from build123d import *

# Parameters (mm, degrees)
SKETCH1_R               = 75
BOSS_EXTRUDE1_DEPTH     = 5
SKETCH2_R               = 14
SKETCH2_R_2             = 10
SKETCH2_R_3             = 4
BOSS_EXTRUDE2_DEPTH     = 25
SKETCH3_R               = 4
CUT_EXTRUDE1_DEPTH      = 12
CUT_EXTRUDE2_REACH      = 122.192
CUT_EXTRUDE2_END_RADIUS = 10
SKETCH4_R               = 1.5
CUT_EXTRUDE3_REACH      = 122.192
CUT_EXTRUDE3_END_RADIUS = 10
SKETCH5_R               = 1.5
SKETCH6_R               = 2
CUT_EXTRUDE4_DEPTH      = 111.227038452
SKETCH7_R               = 1.5
CUT_EXTRUDE5_DEPTH      = 111.227038452
CUT_EXTRUDE6_DEPTH      = 25
BOSS_EXTRUDE3_DEPTH     = 20
SKETCH10_R              = 1.5
CUT_EXTRUDE7_DEPTH      = 113.116290101
FILLET1_R               = 1


with BuildPart() as part:
    # Sketch1 → Boss-Extrude1 (new body)
    with BuildSketch(Plane(origin=(0, 0, 0), x_dir=(1, 0, 0), z_dir=(0, 1, 0))):
        with Locations(Location((0, 0, 0), (0, 0, 270))):
            Circle(SKETCH1_R)
    extrude(amount=BOSS_EXTRUDE1_DEPTH)

    # Sketch2 → Boss-Extrude2 (add)
    with BuildSketch(Plane(origin=(0, 5, 0), x_dir=(1, 0, 0), z_dir=(0, 1, 0))):
        with Locations(Location((0, 0, 0), (0, 0, 270))):
            Circle(SKETCH2_R)
        with Locations(Location((0, 0, 0), (0, 0, 270))):
            Circle(SKETCH2_R_2, mode=Mode.SUBTRACT)
        with Locations(Location((0, 0, 0), (0, 0, 270))):
            Circle(SKETCH2_R_3)
    extrude(amount=BOSS_EXTRUDE2_DEPTH)

    # Sketch3 → Cut-Extrude1 (cut)
    with BuildSketch(Plane(origin=(0, 30, 0), x_dir=(1, 0, 0), z_dir=(0, 1, 0))):
        with Locations(Location((0, 0, 0), (0, 0, 270))):
            Circle(SKETCH3_R)
    extrude(amount=-CUT_EXTRUDE1_DEPTH, mode=Mode.SUBTRACT)

    # Cut-Extrude2: up to this cylinder (the profile starts outside it)
    cut_extrude2_end = Plane(origin=(0, 8.4, 0), z_dir=(0, -1, 0)) * Cylinder(CUT_EXTRUDE2_END_RADIUS, 265.384, mode=Mode.PRIVATE)
    # Sketch4 → Cut-Extrude2 (cut, up to the surface)
    with BuildSketch(Plane(origin=(14, 0, 0), x_dir=(0, 0, -1), z_dir=(1, 0, 0)), mode=Mode.PRIVATE) as cut_extrude2_sk1:
        with Locations((-1, 8.4)):
            Circle(SKETCH4_R)
    cut_extrude2_tool1 = extrude(cut_extrude2_sk1.sketch, amount=-CUT_EXTRUDE2_REACH, mode=Mode.PRIVATE) - cut_extrude2_end
    add(cut_extrude2_tool1.solids().sort_by_distance((14, 8.4, 1))[0], mode=Mode.SUBTRACT)

    # Cut-Extrude3: up to this cylinder (the profile starts outside it)
    cut_extrude3_end = Plane(origin=(0, 8.4, 0), z_dir=(0, -1, 0)) * Cylinder(CUT_EXTRUDE3_END_RADIUS, 265.384, mode=Mode.PRIVATE)
    # Sketch5 → Cut-Extrude3 (cut, up to the surface)
    with BuildSketch(Plane.XY.offset(14), mode=Mode.PRIVATE) as cut_extrude3_sk1:
        with Locations((-1, 8.4)):
            Circle(SKETCH5_R)
    cut_extrude3_tool1 = extrude(cut_extrude3_sk1.sketch, amount=-CUT_EXTRUDE3_REACH, mode=Mode.PRIVATE) - cut_extrude3_end
    add(cut_extrude3_tool1.solids().sort_by_distance((-1, 8.4, 14))[0], mode=Mode.SUBTRACT)

    # Sketch6 → Cut-Extrude4 (cut, through all)
    with BuildSketch(Plane.XZ):
        with Locations(Location((-18, 0, 0), (0, 0, 270))):
            Circle(SKETCH6_R)
        with Locations(Location((18, 0, 0), (0, 0, 270))):
            Circle(SKETCH6_R)
    extrude(amount=-CUT_EXTRUDE4_DEPTH, mode=Mode.SUBTRACT)

    # Sketch7 → Cut-Extrude5 (cut, through all)
    with BuildSketch(Plane.XZ):
        with Locations(Location((20, 47.5, 0), (0, 0, 270))):
            Circle(SKETCH7_R)
        with Locations(Location((33, 47.5, 0), (0, 0, 270))):
            Circle(SKETCH7_R)
        with Locations(Location((20, 25.5, 0), (0, 0, 270))):
            Circle(SKETCH7_R)
        with Locations(Location((33, 25.5, 0), (0, 0, 270))):
            Circle(SKETCH7_R)
        with Locations(Location((-20, 25.5, 0), (0, 0, 270))):
            Circle(SKETCH7_R)
        with Locations(Location((-33, 25.5, 0), (0, 0, 270))):
            Circle(SKETCH7_R)
        with Locations(Location((-33, 47.5, 0), (0, 0, 270))):
            Circle(SKETCH7_R)
        with Locations(Location((-20, 47.5, 0), (0, 0, 270))):
            Circle(SKETCH7_R)
        with Locations(Location((-33, -47.5, 0), (0, 0, 270))):
            Circle(SKETCH7_R)
        with Locations(Location((-20, -47.5, 0), (0, 0, 270))):
            Circle(SKETCH7_R)
        with Locations(Location((-20, -25.5, 0), (0, 0, 270))):
            Circle(SKETCH7_R)
        with Locations(Location((-33, -25.5, 0), (0, 0, 270))):
            Circle(SKETCH7_R)
        with Locations(Location((20, -25.5, 0), (0, 0, 270))):
            Circle(SKETCH7_R)
        with Locations(Location((20, -47.5, 0), (0, 0, 270))):
            Circle(SKETCH7_R)
        with Locations(Location((33, -47.5, 0), (0, 0, 270))):
            Circle(SKETCH7_R)
        with Locations(Location((33, -25.5, 0), (0, 0, 270))):
            Circle(SKETCH7_R)
    extrude(amount=-CUT_EXTRUDE5_DEPTH, mode=Mode.SUBTRACT)

    # Sketch8 → Cut-Extrude6 (cut)
    with BuildSketch(Plane(origin=(0, 30, 0), x_dir=(1, 0, 0), z_dir=(0, 1, 0))):
        with BuildLine():
            Line((0.75, 13.97989628), (0.75, 9.971835338))
            ThreePointArc((0.75, 9.971835338), (0, 10), (-0.75, 9.971835338))
            Line((-0.75, 9.971835338), (-0.75, 13.97989628))
            ThreePointArc((-0.75, 13.97989628), (0, 14), (0.75, 13.97989628))
        make_face()
    extrude(amount=-CUT_EXTRUDE6_DEPTH, mode=Mode.SUBTRACT)

    # Sketch9 → Boss-Extrude3 (add)
    with BuildSketch(Plane(origin=(0, 30, 0), x_dir=(1, 0, 0), z_dir=(0, 1, 0))):
        with BuildLine():
            Line((0.75, 13.97989628), (0.75, 21.727253913))
            Line((0.75, 21.727253913), (2.75, 21.727253913))
            Line((2.75, 21.727253913), (2.75, 13.727253913))
            ThreePointArc((2.75, 13.727253913), (1.754553231, 13.889619972), (0.75, 13.97989628))
        make_face()
        with BuildLine():
            Line((-0.75, 21.727253913), (-2.75, 21.727253913))
            Line((-2.75, 21.727253913), (-2.75, 13.727253913))
            ThreePointArc((-2.75, 13.727253913), (-1.754553231, 13.889619972), (-0.75, 13.97989628))
            Line((-0.75, 13.97989628), (-0.75, 21.727253913))
        make_face()
    extrude(amount=-BOSS_EXTRUDE3_DEPTH)

    # Sketch10 → Cut-Extrude7 (cut, through all)
    with BuildSketch(Plane(origin=(2.75, 0, 0), x_dir=(0, 0, -1), z_dir=(1, 0, 0))):
        with Locations(Location((17.727253913, 24, 0), (0, 0, 180))):
            Circle(SKETCH10_R)
        with Locations(Location((17.727253913, 16, 0), (0, 0, 180))):
            Circle(SKETCH10_R)
    extrude(amount=-CUT_EXTRUDE7_DEPTH, mode=Mode.SUBTRACT)

    # Fillet1
    fillet1_edges = [part.edges().sort_by_distance(p)[0] for p in [
        (13.994973168, 5, 0.375134696),
    ]]
    fillet(fillet1_edges, radius=FILLET1_R)


solid = part.part
Can you work these out from the model? Positions are in its coordinate system, mm. A direction names the side the tool comes from. Round coordinates to 2 decimals unless told otherwise and drop trailing zeros. Write each loop counter-clockwise with the first axis right and the second up, starting at its lowest first coordinate (ties: lowest second). Pieces come first, ordered by that corner, then holes. Notation, with made-up numbers: (25, 31) - (39, 31) arc R18 cw to (39, 52) - close; hole circle Ø2 at (31.25, 78). An arc over 180 degrees is marked (long way). Write each question's results on one line, items separated by ' | '. Start each with the question number.
1) Please list where these lines run through material, in increasing order: line 1 (X direction, y = 1.5, z = 0); line 2 (Z direction, x = -1, y = 16); line 3 (X direction, y = 28.5, z = -16).
2) We'd pull the mould along X, two halves only. Please class faces 4 (the flat face through (-0.75, 20, -16)), 5 (the flat face through (2.75, 20, -18)), 6 (the flat face through (-1, 30, -11)): released by +X, released by -X, zero draft, split by the parting line, or undercut.
3) Suppose I cut it at D-D (z = -42). List the corners of the cut face in (x, y) for me.
4) For pin 1 Ø6 at (y, z) = (15.5, -15.5) entering from +X; pin 2 Ø2.5 at (x, z) = (18, 0) entering from -Y; pin 3 Ø2.5 at (x, y) = (-1, 8.4) entering from +Z; pin 4 Ø4 at (y, z) = (24, -17.73) entering from -X, each with a flat end and sliding along its axis, tell me the tip position at first contact or that it passes through.
5) Suppose I cut it at C-C (x = 59). List the corners of the cut face in (y, z) for me.
6) Which directions (+Z, -Z, +X, -X, +Y, -Y) give clear straight access to the entire face, cutting with the end or side of a thin tool? Please do faces 1 (the cylindrical face through (-3.905, 11.409, -0.867)), 2 (the flat face through (-2.75, 20, -18)), 3 (the flat face through (0.75, 20, -16)).
7) Suppose I cut it at B-B (y = 27.5). List the corners of the cut face in (x, z) for me, and give its area (3 significant figures).
8) Suppose I cut it at A-A (y = 12.5). List the corners of the cut face in (x, z) for me.
Here are the results:
1) line 1: x = -75 to -20, -16 to 16, 20 to 75 | line 2: z = -21.73 to -19.23, -16.23 to -9.95, -3.87 to 3.87, 9.95 to 13.96 | line 3: x = -2.75 to -0.75, 0.75 to 2.75
2) face 4: undercut | face 5: released by +X | face 6: zero draft
3) outline: (-62.14, 0) - (62.14, 0) - (62.14, 5) - (-62.14, 5) - close
4) pin 1: stops at x = 6.3 | pin 2: passes through | pin 3: stops at z = 4 | pin 4: stops at x = -2.75
5) outline: (0, -46.3) - (5, -46.3) - (5, 46.3) - (0, 46.3) - close
6) face 1: +Y | face 2: -Z, -X, +Y | face 3: -Z, +Y
7) outline: (-2.75, -21.73) - (-0.75, -21.73) - (-0.75, -9.97) arc R10 cw (long way) to (0.75, -9.97) - (0.75, -21.73) - (2.75, -21.73) - (2.75, -13.73) arc R14 ccw (long way) to (-2.75, -13.73) - close | area: 327 mm2
8) outline: circle Ø8 at (0, 0); (-2.75, -21.73) - (-0.75, -21.73) - (-0.75, -9.97) arc R10 cw (long way) to (0.75, -9.97) - (0.75, -21.73) - (2.75, -21.73) - (2.75, -13.73) arc R14 ccw (long way) to (-2.75, -13.73) - close
